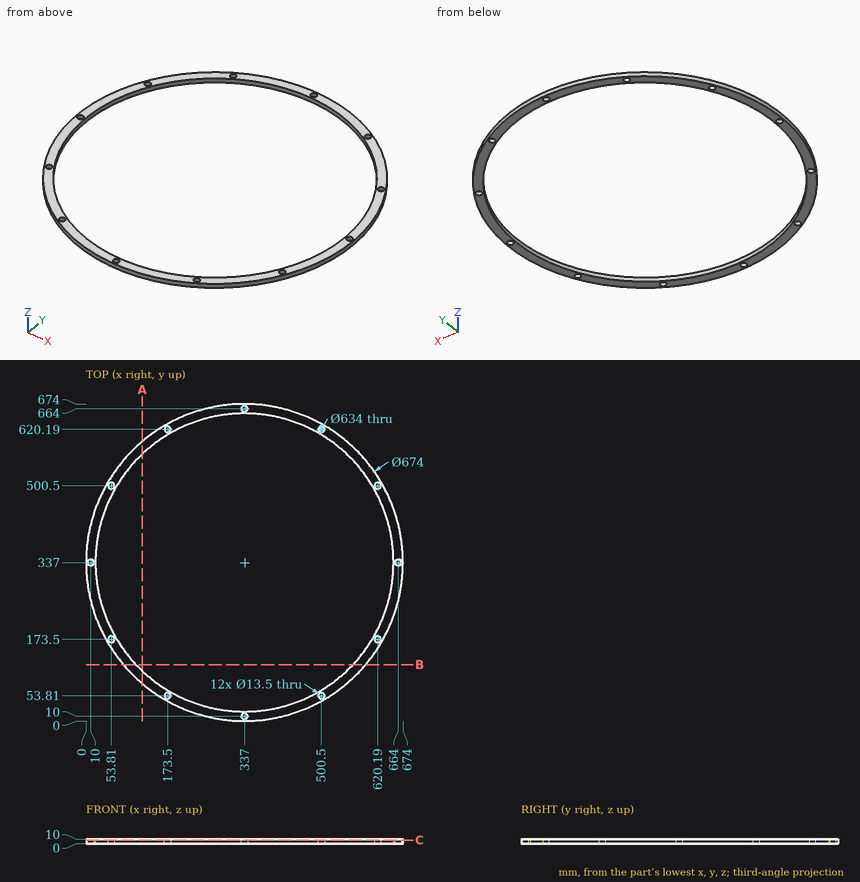
Answer from the drawing. Dimensions are ordinates in mm from the lowest x, y and z of the part. Round coordinates to 2 decimals unless told otherwise and drop trailing zeros. Write each loop counter-clockwise with the first axis right and the second up, starting at its lowest first coordinate (ties: lowest second). Pieces come first, ordered by that corner, then holes. Notation, with made-up numbers: M 78,77.25 L 100,77.25 A16 ccw 100,101.25 Z; hole C 8,-31 d10. An arc over 180 degrees is marked long. Write each question's results on one line, items separated by ' | '. Start each with the question number.
Item 1: A cutting plane is placed at C-C on z = 7.5. State how many separate pieces and enclosed holes the cut face has, and give its area (3 significant figures).
Item 2: A cutting plane is placed at A-A on x = 120. Write down the section's boundary in (y, z) (1 decimal), and give its area (3 significant figures).
Item 3: Straight lines are drawn through the part: L1, parallel to Y at x = 337, z = 2.5; L2, parallel to X at y = 500.5, z = 3.5. For each, find the intervals that lie inside material, in ascending order. Write a range as [from, to].
Item 4: Flat-ended cylindrical pins translate along their axes: pin 1 Ø5 at (x, z) = (307.5, 3) entering from -Y; pin 2 Ø4 at (y, z) = (217, 1.5) entering from -X; pin 3 Ø2 at (y, z) = (496, 7.5) entering from -X. Find the tip coordinate at first contact, or state that the pin passes through.
Check sheet entries:
1) separate pieces: 1 | enclosed holes: 13 | area: 39,400 mm²
2) outline: M 79.2,0 L 105.9,0 L 105.9,10 L 79.2,10 Z; M 568.1,0 L 594.8,0 L 594.8,10 L 568.1,10 Z | area: 535 mm²
3) L1: [0, 3.25], [16.75, 20], [654, 657.25], [670.75, 674] | L2: [42.32, 47.06], [60.56, 65.42], [608.58, 613.44], [626.94, 631.68]
4) pin 1: y = 1.08 | pin 2: x = 21.33 | pin 3: x = 39.33
